Source: CAD feature listing. Evaluate the final solid. Frame: model axes, mm. A direction names the side the tool comes from. Give positions to 0.01 mm unless a question says otherwise; leave off trailing zeros. Loops run counter-clockwise (first coordinate to the right, second up) from the corner with the lowest first, then second, coordinate; pieces in that order, holes last. Notation, with made-up numbers: (-15, 71.5) -> (36, 71.5) arc R20 cw to (36, 107.5) -> close; hole circle Ø11 at (29.5, -28.75). An arc over 180 degrees is marked (long way). Return JSON: item names as keys, results as strings. Group by question number.
(1) Access query for faces 4 (the face through (3, 0, -7)), 5 (the face through (8, 3.556, -5)), 6 (the face through (2.413, 6, -1)), 7 (the face through (9, 6, -7.747)), 8 (the face through (7.096, 1.753, -3.534)). Directions: +Z, -Z, +X, -X, +Y, -Y. A direction counts if a zero-diameter tool reaches every point of the face in a straight line with its end or side. Return the directions, or none.
(2) Ray query, line 1 (Z direction, x = 5.08, y = 1.7); line 2 (Y direction, x = 3.5, z = -3); line 3 (X direction, y = 2.6, z = -5.08). Return the intervals inside material, ascending. Write a range as from..to.
(3) Cut plane A-A on y = 5.75. Return loops of the section in (x, z), then the cut area to 3 significant figures.
(4) Cut plane C-C on x = 5.08. Return loops of the section in (y, z).
(5) Cut plane D-D on y = 3. Return loops of the section in (x, z), then the cut area to 3 significant figures.
(6) Cut plane B-B on z = -5.08. Return loops of the section in (x, y), then the cut area to 3 significant figures.
(7) Draft query along Z for faces 1 (the face through (5, 3, -10.16)), 2 (the face through (5, 10.16, -5)), 3 (the face through (9, 6, -2.413)). Return one class per face: released by +Z, released by -Z, zero draft, split by the parting line, or undercut.
```python
from build123d import *

# Parameters (mm, degrees)
SKETCH2_W           = 10.16
SKETCH2_H           = 10.16
BOSS_EXTRUDE1_DEPTH = 10.16
SKETCH3_R           = 2.54
CUT_EXTRUDE1_DEPTH  = 8.128
CUT_EXTRUDE2_DEPTH  = 10.16
CUT_EXTRUDE3_DEPTH  = 10.16


with BuildPart() as part:
    # Sketch2 → Boss-Extrude1 (new body)
    with BuildSketch(Plane(origin=(0, 0, 0), x_dir=(1, 0, 0), z_dir=(0, 1, 0))):
        with Locations((5.08, 5.08)):
            Rectangle(SKETCH2_W, SKETCH2_H)
    extrude(amount=BOSS_EXTRUDE1_DEPTH)

    # Sketch3 → Cut-Extrude1 (cut)
    with BuildSketch(Plane(origin=(0, 0, 0), x_dir=(-1, 0, 0), z_dir=(0, -1, 0))):
        with Locations((-5.08, 5.08)):
            Circle(SKETCH3_R)
    extrude(amount=-CUT_EXTRUDE1_DEPTH, mode=Mode.SUBTRACT)

    # Sketch6 → Cut-Extrude2 (cut)
    with BuildSketch(Plane(origin=(10.16, 0, 0), x_dir=(0, 0, -1), z_dir=(1, 0, 0))):
        with BuildLine():
            Line((2.921, 8.128), (7.239, 8.128))
            ThreePointArc((7.239, 8.128), (7.598210245, 7.979210245), (7.747, 7.62))
            Line((7.747, 7.62), (7.747, 4.064))
            ThreePointArc((7.747, 4.064), (7.598210245, 3.704789755), (7.239, 3.556))
            Line((7.239, 3.556), (2.921, 3.556))
            ThreePointArc((2.921, 3.556), (2.561789755, 3.704789755), (2.413, 4.064))
            Line((2.413, 4.064), (2.413, 7.62))
            ThreePointArc((2.413, 7.62), (2.561789755, 7.979210245), (2.921, 8.128))
        make_face()
    extrude(amount=-CUT_EXTRUDE2_DEPTH, mode=Mode.SUBTRACT)

    # Sketch4 → Cut-Extrude3 (cut)
    with BuildSketch(Plane.XY):
        with BuildLine():
            Line((2.921, 8.128), (7.239, 8.128))
            ThreePointArc((7.239, 8.128), (7.598210245, 7.979210245), (7.747, 7.62))
            Line((7.747, 7.62), (7.747, 4.064))
            ThreePointArc((7.747, 4.064), (7.598210245, 3.704789755), (7.239, 3.556))
            Line((7.239, 3.556), (2.921, 3.556))
            ThreePointArc((2.921, 3.556), (2.561789755, 3.704789755), (2.413, 4.064))
            Line((2.413, 4.064), (2.413, 7.62))
            ThreePointArc((2.413, 7.62), (2.561789755, 7.979210245), (2.921, 8.128))
        make_face()
    extrude(amount=-CUT_EXTRUDE3_DEPTH, mode=Mode.SUBTRACT)


solid = part.part
```
Answers:
{
 "1": {"face 4": "+Z, -Z, +X, -X, -Y", "face 5": "none", "face 6": "+Z, -Z", "face 7": "+X, -X", "face 8": "-Y"},
 "2": {"line 1": "-10.16..-7.62, -2.54..0", "line 2": "0..3.56, 8.13..10.16", "line 3": "0..2.54, 7.62..10.16"},
 "3": {"outline": "(0, -10.16) -> (2.41, -10.16) -> (2.41, -7.75) -> (0, -7.75) -> close; (0, -2.41) -> (2.41, -2.41) -> (2.41, 0) -> (0, 0) -> close; (7.75, -10.16) -> (10.16, -10.16) -> (10.16, -7.75) -> (7.75, -7.75) -> close; (7.75, -2.41) -> (10.16, -2.41) -> (10.16, 0) -> (7.75, 0) -> close", "area": "23.3 mm²"},
 "4": {"outline": "(0, -10.16) -> (3.56, -10.16) -> (3.56, -7.62) -> (0, -7.62) -> close; (0, -2.54) -> (3.56, -2.54) -> (3.56, 0) -> (0, 0) -> close; (8.13, -10.16) -> (10.16, -10.16) -> (10.16, 0) -> (8.13, 0) -> close"},
 "5": {"outline": "(0, -10.16) -> (10.16, -10.16) -> (10.16, 0) -> (0, 0) -> close; hole circle Ø5.08 at (5.08, -5.08)", "area": "83.0 mm²"},
 "6": {"outline": "(0, 0) -> (2.54, 0) -> (2.54, 3.56) -> (0, 3.56) -> close; (0, 8.13) -> (10.16, 8.13) -> (10.16, 10.16) -> (0, 10.16) -> close; (7.62, 0) -> (10.16, 0) -> (10.16, 3.56) -> (7.62, 3.56) -> close", "area": "38.7 mm²"},
 "7": {"face 1": "released by -Z", "face 2": "zero draft", "face 3": "undercut"}
}
